Part model, mm, in its own coordinate system. Face numbers are marked on the shaded views. A direction names the side the tool comes from. Give positions to 0.01 mm unless a question says otherwise; leave off trailing zeros. Write each loop counter-clockwise with the first axis right and the second up, starting at its lowest first coordinate (ties: lowest second). Pieces come first, ordered by that corner, then holes.
```python
from build123d import *

# Parameters (mm, degrees)
SKETCH1_W           = 50.8
SKETCH1_H           = 50.8
SKETCH1_W_2         = 44.416753927
SKETCH1_H_2         = 44.416753927
BOSS_EXTRUDE1_DEPTH = 177.8
SKETCH2_R           = 6.35
CUT_EXTRUDE1_DEPTH  = 51.8


with BuildPart() as part:
    # Sketch1 → Boss-Extrude1 (new body)
    with BuildSketch(Plane(origin=(0, 0, 0), x_dir=(1, 0, 0), z_dir=(0, 1, 0))):
        Rectangle(SKETCH1_W, SKETCH1_H)
        with Locations((-0.016623037, 0.016623037)):
            Rectangle(SKETCH1_W_2, SKETCH1_H_2, mode=Mode.SUBTRACT)
    extrude(amount=BOSS_EXTRUDE1_DEPTH)

    # Sketch2 → Cut-Extrude1 (cut, through all)
    with BuildSketch(Plane.ZY.offset(25.4)):
        with Locations((0, 25.4)):
            Circle(SKETCH2_R)
        with Locations((0, 152.4)):
            Circle(SKETCH2_R)
    extrude(amount=-CUT_EXTRUDE1_DEPTH, mode=Mode.SUBTRACT)


solid = part.part
```
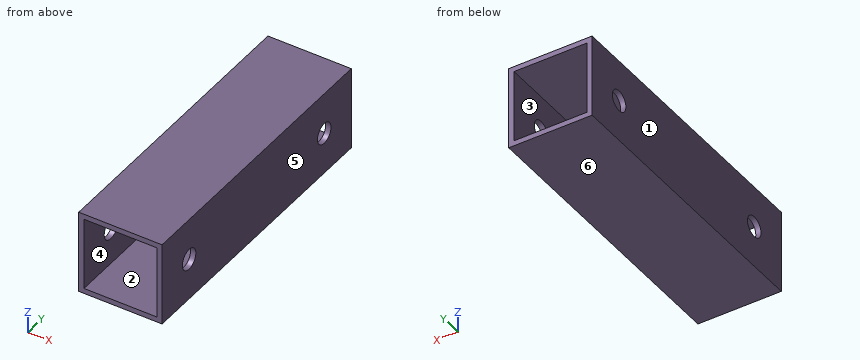
1) Saw through at C-C, the plane x = -11.5. Write the cut outline in (y, z) (3 decimals), then the cut area to 3 significant figures.
Answers follow:
outline: (0, -25.4) - (177.8, -25.4) - (177.8, -22.225) - (0, -22.225) - close; (0, 22.192) - (177.8, 22.192) - (177.8, 25.4) - (0, 25.4) - close
area: 1,130 mm2
2) 3-axis set-ups, long thin cutter, end or side, ignore diameter. For the marked faces 1 and 2: which of +Z, -Z, +X, -X, +Y, -Y reach the whole face in a straight line?
Answers follow:
face 1: +Z, -Z, -X, +Y, -Y
face 2: +Y, -Y
3) Two-plate mould, pull along X, no slides. Class the marked faces 3, 4, 5 and 6: +X half, -X half, draft (parallel to the pull), parting line (faces both ways), or undercut.
Answers follow:
face 3: undercut
face 4: undercut
face 5: +X half
face 6: draft
4) Saw through at D-D, the plane y = 25.4. Write the cut outline in (x, z) (3 decimals).
Answers follow:
outline: (-25.4, -25.4) - (25.4, -25.4) - (25.4, -6.35) - (22.192, -6.35) - (22.192, -22.225) - (-22.225, -22.225) - (-22.225, -6.35) - (-25.4, -6.35) - close; (-25.4, 6.35) - (-22.225, 6.35) - (-22.225, 22.192) - (22.192, 22.192) - (22.192, 6.35) - (25.4, 6.35) - (25.4, 25.4) - (-25.4, 25.4) - close
5) Wall check: L1, parallel to Y at x = -24.35, z = 0; L2, parallel to Z at x = -21, y = 16.5 (3 decimals). Give the ranges that are in metal, low to high.
Answers follow:
L1: y = 0 to 19.05, 31.75 to 146.05, 158.75 to 177.8
L2: z = -25.4 to -22.225, 22.192 to 25.4
6) Saw through at A-A, the plane y = 84. Write the cut outline in (x, z) (3 decimals), then the cut area to 3 significant figures.
Answers follow:
outline: (-25.4, -25.4) - (25.4, -25.4) - (25.4, 25.4) - (-25.4, 25.4) - close; hole (-22.225, -22.225) - (22.192, -22.225) - (22.192, 22.192) - (-22.225, 22.192) - close
area: 608 mm2
7) Saw through at B-B, the plane z = 0. Write the cut outline in (x, y) (3 decimals), then the cut area to 3 significant figures.
Answers follow:
outline: (-25.4, 0) - (-22.225, 0) - (-22.225, 19.05) - (-25.4, 19.05) - close; (-25.4, 31.75) - (-22.225, 31.75) - (-22.225, 146.05) - (-25.4, 146.05) - close; (-25.4, 158.75) - (-22.225, 158.75) - (-22.225, 177.8) - (-25.4, 177.8) - close; (22.192, 0) - (25.4, 0) - (25.4, 19.05) - (22.192, 19.05) - close; (22.192, 31.75) - (25.4, 31.75) - (25.4, 146.05) - (22.192, 146.05) - close; (22.192, 158.75) - (25.4, 158.75) - (25.4, 177.8) - (22.192, 177.8) - close
area: 973 mm2
